Read the model definition and answer for the solid it produces. Units are mm, in the model's axes. A direction names the side the tool comes from. Round coordinates to 2 decimals unless told otherwise and drop trailing zeros. Write each loop counter-clockwise with the first axis right and the second up, starting at its lowest first coordinate (ties: lowest second). Pieces come first, ordered by that corner, then holes. Notation, with made-up numbers: (-26.5, 11.5) -> (6.5, 11.5) arc R28 ccw to (6.5, 44.5) -> close; hole circle Ø10 at (11.25, 33). An arc over 180 degrees is marked (long way). Return JSON: item names as keys, results as strings.
from build123d import *

# Parameters (mm, degrees)
F1_DEPTH = 25.4


with BuildPart() as f1:
    # F0 (on Front) → F1 (new body)
    with BuildSketch(Plane.XZ):
        Polygon((-69.6489065795, 213.2151687083), (-192.2873854637, 44.417783618), (-69.6489065795, -124.3796014723), (128.7843205837, -59.9047375799), (128.7843205837, 148.7403048159), align=None)
        with BuildLine():
            Line((-113.6227780141, -5.6910817596), (-113.6227780141, 8.5026193143))
            Line((-113.6227780141, 8.5026193143), (-81.7353182283, 8.5026193143))
            Line((-81.7353182283, 8.5026193143), (-81.7353182283, -33.1638959821))
            add(Edge.make_bspline(
                [(-81.7353182283, -33.1638959821), (-89.4917273654, -35.6966010064), (-96.333548577, -36.7167183079)],
                knots=[0, 0, 0, 1, 1, 1], degree=2))
            add(Edge.make_bspline(
                [(-96.333548577, -36.7167183079), (-103.1753697886, -37.7368356094), (-110.3161908989, -37.7368356094)],
                knots=[0, 0, 0, 1, 1, 1], degree=2))
            add(Edge.make_bspline(
                [(-110.3161908989, -37.7368356094), (-128.5024200321, -37.7368356094), (-138.0967991348, -27.0431921732)],
                knots=[0, 0, 0, 1, 1, 1], degree=2))
            add(Edge.make_bspline(
                [(-138.0967991348, -27.0431921732), (-147.6911782374, -16.3495487371), (-147.6911782374, 3.665856247)],
                knots=[0, 0, 0, 1, 1, 1], degree=2))
            add(Edge.make_bspline(
                [(-147.6911782374, 3.665856247), (-147.6911782374, 23.1184378924), (-136.5578290679, 33.9967577365)],
                knots=[0, 0, 0, 1, 1, 1], degree=2))
            add(Edge.make_bspline(
                [(-136.5578290679, 33.9967577365), (-125.4244798984, 44.8750775807), (-105.708074813, 44.8750775807)],
                knots=[0, 0, 0, 1, 1, 1], degree=2))
            add(Edge.make_bspline(
                [(-105.708074813, 44.8750775807), (-93.3259613606, 44.8750775807), (-81.8408476043, 39.9327851374)],
                knots=[0, 0, 0, 1, 1, 1], degree=2))
            Line((-81.8408476043, 39.9327851374), (-87.5042574504, 26.3019074021))
            add(Edge.make_bspline(
                [(-87.5042574504, 26.3019074021), (-96.2983721183, 30.6989647361), (-105.813604189, 30.6989647361)],
                knots=[0, 0, 0, 1, 1, 1], degree=2))
            add(Edge.make_bspline(
                [(-105.813604189, 30.6989647361), (-116.8590122118, 30.6989647361), (-123.5073629008, 23.2767319564)],
                knots=[0, 0, 0, 1, 1, 1], degree=2))
            add(Edge.make_bspline(
                [(-123.5073629008, 23.2767319564), (-130.1557135897, 15.8544991767), (-130.1557135897, 3.3316798896)],
                knots=[0, 0, 0, 1, 1, 1], degree=2))
            add(Edge.make_bspline(
                [(-130.1557135897, 3.3316798896), (-130.1557135897, -9.7539627362), (-124.8000977569, -16.6485486358)],
                knots=[0, 0, 0, 1, 1, 1], degree=2))
            add(Edge.make_bspline(
                [(-124.8000977569, -16.6485486358), (-119.4444819242, -23.5431345354), (-109.2257206801, -23.5431345354)],
                knots=[0, 0, 0, 1, 1, 1], degree=2))
            add(Edge.make_bspline(
                [(-109.2257206801, -23.5431345354), (-103.878898962, -23.5431345354), (-98.3913714093, -22.4526643166)],
                knots=[0, 0, 0, 1, 1, 1], degree=2))
            Line((-98.3913714093, -22.4526643166), (-98.3913714093, -5.6910817596))
            Line((-98.3913714093, -5.6910817596), (-113.6227780141, -5.6910817596))
        make_face(mode=Mode.SUBTRACT)
        with BuildLine():
            add(Edge.make_bspline(
                [(-23.9228084016, -36.6639536199), (-28.917865533, -37.7368356094), (-36.1290395607, -37.7368356094)],
                knots=[0, 0, 0, 1, 1, 1], degree=2))
            add(Edge.make_bspline(
                [(-36.1290395607, -37.7368356094), (-50.9559168907, -37.7368356094), (-59.3103258252, -29.5407207389)],
                knots=[0, 0, 0, 1, 1, 1], degree=2))
            add(Edge.make_bspline(
                [(-59.3103258252, -29.5407207389), (-67.6647347597, -21.3446058685), (-67.6647347597, -6.341846245)],
                knots=[0, 0, 0, 1, 1, 1], degree=2))
            add(Edge.make_bspline(
                [(-67.6647347597, -6.341846245), (-67.6647347597, 9.1006191118), (-59.9435020813, 17.5341750783)],
                knots=[0, 0, 0, 1, 1, 1], degree=2))
            add(Edge.make_bspline(
                [(-59.9435020813, 17.5341750783), (-52.2222694029, 25.9677310448), (-38.5913916677, 25.9677310448)],
                knots=[0, 0, 0, 1, 1, 1], degree=2))
            add(Edge.make_bspline(
                [(-38.5913916677, 25.9677310448), (-25.5761019592, 25.9677310448), (-18.3209573582, 18.5542923797)],
                knots=[0, 0, 0, 1, 1, 1], degree=2))
            add(Edge.make_bspline(
                [(-18.3209573582, 18.5542923797), (-11.0658127572, 11.1408537147), (-11.0658127572, -1.9447889111)],
                knots=[0, 0, 0, 1, 1, 1], degree=2))
            Line((-11.0658127572, -1.9447889111), (-11.0658127572, -10.0881390936))
            Line((-11.0658127572, -10.0881390936), (-50.6920934507, -10.0881390936))
            add(Edge.make_bspline(
                [(-50.6920934507, -10.0881390936), (-50.4106817813, -17.2289602039), (-46.4533301808, -21.2390764924)],
                knots=[0, 0, 0, 1, 1, 1], degree=2))
            add(Edge.make_bspline(
                [(-46.4533301808, -21.2390764924), (-42.4959785802, -25.249192781), (-35.3551574699, -25.249192781)],
                knots=[0, 0, 0, 1, 1, 1], degree=2))
            add(Edge.make_bspline(
                [(-35.3551574699, -25.249192781), (-29.7972769998, -25.249192781), (-24.8549845564, -24.0971637595)],
                knots=[0, 0, 0, 1, 1, 1], degree=2))
            add(Edge.make_bspline(
                [(-24.8549845564, -24.0971637595), (-19.9126921131, -22.945134738), (-14.5306939363, -20.4124297137)],
                knots=[0, 0, 0, 1, 1, 1], degree=2))
            Line((-14.5306939363, -20.4124297137), (-14.5306939363, -33.3925429635))
            add(Edge.make_bspline(
                [(-14.5306939363, -33.3925429635), (-18.9277512703, -35.5910716304), (-23.9228084016, -36.6639536199)],
                knots=[0, 0, 0, 1, 1, 1], degree=2))
        make_face(mode=Mode.SUBTRACT)
        with BuildLine():
            Line((34.3821718464, -36.6287771612), (17.180883556, -36.6287771612))
            Line((17.180883556, -36.6287771612), (-6.2290496899, 24.8244961379))
            Line((-6.2290496899, 24.8244961379), (11.3064149579, 24.8244961379))
            Line((11.3064149579, 24.8244961379), (23.1784697595, -10.1936684696))
            add(Edge.make_bspline(
                [(23.1784697595, -10.1936684696), (25.1483514451, -16.8420191585), (25.6584100959, -22.7692524447)],
                knots=[0, 0, 0, 1, 1, 1], degree=2))
            Line((25.6584100959, -22.7692524447), (25.9749982239, -22.7692524447))
            add(Edge.make_bspline(
                [(25.9749982239, -22.7692524447), (26.2564098933, -17.4927836439), (28.4549385603, -10.1936684696)],
                knots=[0, 0, 0, 1, 1, 1], degree=2))
            Line((28.4549385603, -10.1936684696), (40.2742286739, 24.8244961379))
            Line((40.2742286739, 24.8244961379), (57.8096933217, 24.8244961379))
            Line((57.8096933217, 24.8244961379), (34.3821718464, -36.6287771612))
        make_face(mode=Mode.SUBTRACT)
        with BuildLine():
            Line((117.3282613939, -36.6287771612), (105.6320888856, -36.6287771612))
            Line((105.6320888856, -36.6287771612), (102.3782664585, -28.2743682268))
            Line((102.3782664585, -28.2743682268), (101.9385607251, -28.2743682268))
            add(Edge.make_bspline(
                [(101.9385607251, -28.2743682268), (97.7173856845, -33.6036017155), (93.2323872039, -35.6702186624)],
                knots=[0, 0, 0, 1, 1, 1], degree=2))
            add(Edge.make_bspline(
                [(93.2323872039, -35.6702186624), (88.7473887233, -37.7368356094), (81.5538029249, -37.7368356094)],
                knots=[0, 0, 0, 1, 1, 1], degree=2))
            add(Edge.make_bspline(
                [(81.5538029249, -37.7368356094), (72.7069235691, -37.7368356094), (67.623925291, -32.6714255607)],
                knots=[0, 0, 0, 1, 1, 1], degree=2))
            add(Edge.make_bspline(
                [(67.623925291, -32.6714255607), (62.540927013, -27.606015512), (62.540927013, -18.2666657347)],
                knots=[0, 0, 0, 1, 1, 1], degree=2))
            add(Edge.make_bspline(
                [(62.540927013, -18.2666657347), (62.540927013, -8.487610224), (69.3827482246, -3.8443176794)],
                knots=[0, 0, 0, 1, 1, 1], degree=2))
            add(Edge.make_bspline(
                [(69.3827482246, -3.8443176794), (76.2245694362, 0.7989748653), (90.0137412355, 1.2914452867)],
                knots=[0, 0, 0, 1, 1, 1], degree=2))
            Line((90.0137412355, 1.2914452867), (100.6897964423, 1.6256216441))
            Line((100.6897964423, 1.6256216441), (100.6897964423, 4.3166207324))
            add(Edge.make_bspline(
                [(100.6897964423, 4.3166207324), (100.6897964423, 13.6559705097), (91.1217996836, 13.6559705097)],
                knots=[0, 0, 0, 1, 1, 1], degree=2))
            add(Edge.make_bspline(
                [(91.1217996836, 13.6559705097), (83.7523315919, 13.6559705097), (73.7973937879, 9.2061484878)],
                knots=[0, 0, 0, 1, 1, 1], degree=2))
            Line((73.7973937879, 9.2061484878), (68.2571015471, 20.53296818))
            add(Edge.make_bspline(
                [(68.2571015471, 20.53296818), (78.8628038366, 26.0908486501), (91.772564169, 26.0908486501)],
                knots=[0, 0, 0, 1, 1, 1], degree=2))
            add(Edge.make_bspline(
                [(91.772564169, 26.0908486501), (104.1370893921, 26.0908486501), (110.732675393, 20.7000563587)],
                knots=[0, 0, 0, 1, 1, 1], degree=2))
            add(Edge.make_bspline(
                [(110.732675393, 20.7000563587), (117.3282613939, 15.3092640673), (117.3282613939, 4.3166207324)],
                knots=[0, 0, 0, 1, 1, 1], degree=2))
            Line((117.3282613939, 4.3166207324), (117.3282613939, -36.6287771612))
        make_face(mode=Mode.SUBTRACT)
    extrude(amount=F1_DEPTH)


solid = f1.part
Item 1: Section D-D (x = -160.5) is taken. Give the vertices of the cut face in (y, z).
Worked answers:
{"outline": "(-25.4, 0.67) -> (0, 0.67) -> (0, 88.17) -> (-25.4, 88.17) -> close"}
Item 2: Section A-A (x = 46) is taken. Give the vertices of the cut face in (y, z), then the cut area to 3 significant figures.
Worked answers:
{"outline": "(-25.4, -86.8) -> (0, -86.8) -> (0, -6.15) -> (-25.4, -6.15) -> close; (-25.4, 24.82) -> (0, 24.82) -> (0, 175.64) -> (-25.4, 175.64) -> close", "area": "5,880 mm2"}
Item 3: For a pull along Z with two mould halves and no side action, classify faces 1 (the flat face through (-84.633, -12.522, 33.213)), 2 (the flat face through (-130.11, -12.52, 130)), 3 (the flat face through (2, -13, 24.824)), 4 (the flat face through (-131.827, -12.522, -38.799)) as released by +Z, released by -Z, zero draft, split by the parting line, or undercut.
Worked answers:
{"face 1": "undercut", "face 2": "released by +Z", "face 3": "undercut", "face 4": "released by -Z"}
Item 4: Section C-C (z = 166) is taken. Give the vertices of the cut face in (x, y).
Worked answers:
{"outline": "(-103.95, -25.4) -> (75.66, -25.4) -> (75.66, 0) -> (-103.95, 0) -> close"}
Item 5: Straight lines are drawn through the part: L1, parallel to Z at x = -16.5, y = -9.75; L2, parallel to Z at x = -109.5, y = -20.5; L3, parallel to Z at x = 78.5, y = -2.25. For each, find the intervals that lie inside material, in ascending order. Write a range as [from, to].
Worked answers:
{"L1": "z = [-107.11, -34.31], [-21.3, -10.09], [16.46, 195.95]", "L2": "z = [-69.53, -37.73], [-23.54, -5.69], [8.5, 30.48], [44.77, 158.36]", "L3": "z = [-76.24, -37.57], [-0.11, 11.11], [24.47, 165.08]"}
Item 6: A tool of negligible diameter and unlimited length cuts with its end or side. For faces 5 (the flat face through (-34, -25.4, 47)), 6 (the flat face through (-14.531, -13, -27)), from which of +Z, -Z, +X, -X, +Y, -Y can it reach the whole face along a straight path? Write none if from no direction.
Worked answers:
{"face 5": "+Z, -Z, +X, -X, -Y", "face 6": "+Y, -Y"}
Item 7: Flat-ended cylindrical pins translate along their axes: pin 1 (4 mm diameter, centred on y = -9.5, z = -25, fed in from -X); pin 2 (5 mm diameter, centred on y = -17, z = -17, fed in from -X); pin 3 (12.5 mm diameter, centred on y = -17, z = -7.5, fed in from -X). Find the tip coordinate at first contact, or state that the pin passes through.
Worked answers:
{"pin 1": "stops at x = -143.31", "pin 2": "stops at x = -149.48", "pin 3": "stops at x = -159.11"}
Item 8: Section B-B (y = -12.5) is taken. State how many separate pieces and enclosed holes the cut face has, then the cut area to 3 significant figures.
Worked answers:
{"separate pieces": "1", "enclosed holes": "4", "area": "64,800 mm2"}
